Input: part model. Units: mm. Frame: model coordinates. A direction names the side the tool comes from. Coordinates: 2 decimals unless noted, no trailing zeros. Write each loop counter-clockwise with the first axis right and the second up, starting at its lowest first coordinate (ties: lowest second). Pieces come first, ordered by that corner, then holes.
1) Draft query along Y for faces 6 (the flat face through (-11, -4.265, 9)), 7 (the cylindrical face through (25.385, -12.86, 2.535)), 8 (the flat face through (27, 0.735, 6)). Return one class per face: pulls with the +Y half, pulls with the -Y half, needs draft (parallel to the pull), parting line crosses it, or undercut.
2) Pin query (flat end, axial travel): pin 1 Ø2.5 at (y, z) = (-0.5, 8.5) entering from +X; pin 2 Ø6 at (x, y) = (0.5, -7) entering from -Z; pin 3 Ø3 at (x, y) = (-14, 4) entering from +Z; pin 4 Ø4 at (x, z) = (23, 8) entering from -Y. Return the tip coordinate at first contact, or that it passes through.
3) Set-up query: faces 1 (the flat face through (34.214, -2, 6)), 2 (the flat face through (-0.686, 6, 9)), 3 (the flat face through (-5.686, 8, 6)), 4 (the flat face through (18, 1, 12.45)), 5 (the flat face through (24, -4.265, 9)). Return all of +Z, -Z, +X, -X, +Y, -Y with unobstructed straight access to the full face (end or side cutting, diameter ignored); none if empty.
4) Section query D-D (y = -11). Output: boundary loops of the cut face in (x, z), then the cut area to 3 significant figures.
5) Section query A-A (z = 7.5). Output: boundary loops of the cut face in (x, y), then the cut area to 3 significant figures.
6) Section query C-C (x = 6.5). Output: boundary loops of the cut face in (y, z), then the cut area to 3 significant figures.
7) Section query B-B (y = 0). Output: boundary loops of the cut face in (x, z), then the cut area to 4 significant figures.
8) Line query: L1, parallel to X at y = -13, z = 3.75; L2, parallel to X at y = 5, z = 8; L3, parallel to X at y = -2, z = 5.25. Output: solid intervals per line, ascending.
from build123d import *

# Parameters (mm, degrees)
BOSS_EXTRUDE1_DEPTH = 5
BOSS_EXTRUDE2_DEPTH = 12.45
SKETCH6_R           = 1.8
CUT_EXTRUDE3_DEPTH  = 6


with BuildPart() as part:
    # Sketch1 → Boss-Extrude1 (new body)
    with BuildSketch(Plane.XY):
        Polygon((14.31372549, -4.264705882), (34.31372549, -4.264705882), (34.31372549, -19.264705882), (-20.68627451, -19.264705882), (-20.68627451, -4.264705882), (-0.68627451, -4.264705882), (-0.68627451, 15.735294118), (14.31372549, 15.735294118), align=None)
    extrude(amount=BOSS_EXTRUDE1_DEPTH)

    # Sketch2 → Boss-Extrude2 (add)
    with BuildSketch(Plane(origin=(0, 0, 0), x_dir=(-1, 0, 0), z_dir=(0, 0, -1))):
        Polygon((0.68627451, 15.735294118), (5.68627451, 15.735294118), (5.68627451, 0.735294118), (6.079970528, 0.735294118), (20.68627451, 0.735294118), (20.68627451, -4.264705882), (0.68627451, -4.264705882), align=None)
    boss_extrude2 = extrude(amount=-BOSS_EXTRUDE2_DEPTH)

    # Mirror1: Boss-Extrude2 across plane
    add(boss_extrude2.mirror(Plane.ZY.offset(-6.76372549)))

    # Sketch6 → Cut-Extrude3 (cut, through all)
    with BuildSketch(Plane.XY.offset(5)):
        with Locations((6.76372549, 8.235294118)):
            Circle(SKETCH6_R)
        with Locations((-13.18627451, -11.764705882)):
            Circle(SKETCH6_R)
        with Locations((26.81372549, -11.764705882)):
            Circle(SKETCH6_R)
    extrude(amount=-CUT_EXTRUDE3_DEPTH, mode=Mode.SUBTRACT)


solid = part.part
Answer:
1. face 6: pulls with the -Y half
1. face 7: undercut
1. face 8: pulls with the +Y half
2. pin 1: stops at x = 34.21
2. pin 2: stops at z = 0
2. pin 3: passes through
2. pin 4: stops at y = -4.26
3. face 1: +Z, -Z, +X, +Y
3. face 2: +Z, +Y, -Y
3. face 3: +Z, -Z, -X, +Y
3. face 4: +Z, +X, -X, +Y, -Y
3. face 5: +Z, +X, -X, -Y
4. outline: (-20.69, 0) - (-14.82, 0) - (-14.82, 5) - (-20.69, 5) - close; (-11.56, 0) - (25.18, 0) - (25.18, 5) - (-11.56, 5) - close; (28.44, 0) - (34.31, 0) - (34.31, 5) - (28.44, 5) - close
4. area: 242 mm2
5. outline: (-20.69, -4.26) - (-0.69, -4.26) - (-0.69, 15.74) - (-5.69, 15.74) - (-5.69, 0.74) - (-20.69, 0.74) - close; (14.21, -4.26) - (34.21, -4.26) - (34.21, 0.74) - (19.21, 0.74) - (19.21, 15.74) - (14.21, 15.74) - close
5. area: 350 mm2
6. outline: (-19.26, 0) - (6.45, 0) - (6.45, 5) - (-19.26, 5) - close; (10.02, 0) - (15.74, 0) - (15.74, 5) - (10.02, 5) - close
6. area: 157 mm2
7. outline: (-20.69, 0) - (34.21, 0) - (34.21, 12.45) - (14.21, 12.45) - (14.21, 5) - (-0.69, 5) - (-0.69, 12.45) - (-20.69, 12.45) - close
7. area: 572.5 mm2
8. L1: x = -20.69 to -14.5, -11.88 to 25.5, 28.12 to 34.31
8. L2: x = -5.69 to -0.69, 14.21 to 19.21
8. L3: x = -20.69 to -0.69, 14.21 to 34.21
